Work out the finished part from the listing and answer in its coordinate system (mm). Face numbers are marked on the shaded views. A direction names the side the tool comes from. Round coordinates to 2 decimals unless told otherwise and drop trailing zeros. Order: outer loops, then holes, each group sorted by start corner. A loop starts at its lowest first (then second) coordinate and runs counter-clockwise, first axis right, second up. Notation, with made-up numbers: M 16,31 L 28,31 A16 ccw 28,57 Z; hole C 62,4 d1. An arc over 180 degrees is marked long. Return JSON: item names as keys, results as strings.
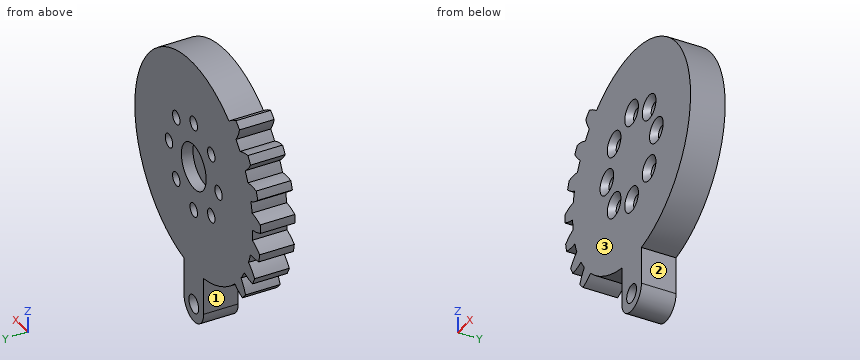
from build123d import *

# Parameters (mm, degrees)
SKETCH1_R                                       = 19.05
BOSS_EXTRUDE1_DEPTH                             = 6
SKETCH8_R                                       = 4
CUT_EXTRUDE4_DEPTH                              = 2
BOSS_EXTRUDE3_DEPTH                             = 6
CIRPATTERN2_DEPTH                               = 6
SKETCH4_R                                       = 1.5875
BOSS_EXTRUDE4_DEPTH                             = 6
CSK_FOR_M2_FLAT_HEAD_MACHINE_SCREW1_D           = 2.4
CSK_FOR_M2_FLAT_HEAD_MACHINE_SCREW1_CSINK_D     = 4.4
CSK_FOR_M2_FLAT_HEAD_MACHINE_SCREW1_CSINK_ANGLE = 90
CIRPATTERN3_COUNT                               = 8


# Read off the part's stored shape, not the designer's step: CirPattern2
with BuildPart() as part:
    # Sketch1 → Boss-Extrude1 (new body)
    with BuildSketch(Plane(origin=(0, 0, 0), x_dir=(1, 0, 0), z_dir=(0, 1, 0))):
        with Locations(Location((0, 0, 0), (0, 0, 270))):
            Circle(SKETCH1_R)
    extrude(amount=BOSS_EXTRUDE1_DEPTH)

    # Sketch8 → Cut-Extrude4 (cut)
    with BuildSketch(Plane.XZ.offset(-6)):
        with Locations(Location((0, 0, 0), (0, 0, 270))):
            Circle(SKETCH8_R)
    extrude(amount=CUT_EXTRUDE4_DEPTH, mode=Mode.SUBTRACT)

    # Sketch3 → Boss-Extrude3 (add)
    with BuildSketch(Plane(origin=(0, 0, 0), x_dir=(1, 0, 0), z_dir=(0, 1, 0))):
        with BuildLine():
            ThreePointArc((-18.32709122, 5.198098444), (-19.680979383, 5.197152008), (-21.013329851, 4.956618665))
            ThreePointArc((-21.013329851, 4.956618665), (-21.175154204, 4.212000052), (-21.310601203, 3.462134657))
            ThreePointArc((-21.310601203, 3.462134657), (-20.171718001, 2.730042376), (-18.921250622, 2.211057413))
            ThreePointArc((-18.921250622, 2.211057413), (-18.683959592, 3.716470634), (-18.32709122, 5.198098444))
        make_face()
    extrude(amount=BOSS_EXTRUDE3_DEPTH)

    # CirPattern2 outline → CirPattern2 (add)
    with BuildSketch(Plane(origin=(0, 0, 0), x_dir=(1, 0, 0), z_dir=(0, 1, 0))):
        with BuildLine():
            ThreePointArc((-17.704260875, 7.032897477), (-17.085425728, 8.425599549), (-16.357243856, 9.764377784))
            ThreePointArc((-16.357243856, 9.764377784), (-17.665244353, 10.113875638), (-19.014450689, 10.226375946))
            ThreePointArc((-19.014450689, 10.226375946), (-19.36348249, 9.549012822), (-19.688393689, 8.859754733))
            ThreePointArc((-19.688393689, 8.859754733), (-18.777796417, 7.857843228), (-17.704260875, 7.032897477))
        make_face()
        with BuildLine():
            ThreePointArc((-15.280755006, 11.375457202), (-14.322548335, 12.560537779), (-13.272677354, 13.665230916))
            ThreePointArc((-13.272677354, 13.665230916), (-14.445652113, 14.341355358), (-15.719768136, 14.799222606))
            ThreePointArc((-15.719768136, 14.799222606), (-16.232221443, 14.235276148), (-16.724454683, 13.653597166))
            ThreePointArc((-16.724454683, 13.653597166), (-16.104199039, 12.450145051), (-15.280755006, 11.375457202))
        make_face()
        with BuildLine():
            ThreePointArc((-11.375457197, -15.280755), (-12.560537774, -14.322548329), (-13.66523091, -13.272677349))
            ThreePointArc((-13.66523091, -13.272677349), (-14.341355358, -14.445652113), (-14.799222606, -15.719768136))
            ThreePointArc((-14.799222606, -15.719768136), (-14.235276148, -16.232221443), (-13.653597166, -16.724454683))
            ThreePointArc((-13.653597166, -16.724454683), (-12.450145051, -16.104199039), (-11.375457197, -15.280755))
        make_face()
        with BuildLine():
            ThreePointArc((-14.942798311, -11.81589093), (-15.839496111, -10.583612937), (-16.634821136, -9.28359982))
            ThreePointArc((-16.634821136, -9.28359982), (-17.59149541, -10.241612555), (-18.363526703, -11.353809363))
            ThreePointArc((-18.363526703, -11.353809363), (-17.95142893, -11.994761331), (-17.516969515, -12.620771728))
            ThreePointArc((-17.516969515, -12.620771728), (-16.193990063, -12.33312711), (-14.942798311, -11.81589093))
        make_face()
        with BuildLine():
            ThreePointArc((-17.491812414, -7.545793421), (-18.039018964, -6.123421813), (-18.470775793, -4.661860306))
            ThreePointArc((-18.470775793, -4.661860306), (-19.642804121, -5.339624026), (-20.676386801, -6.214107244))
            ThreePointArc((-20.676386801, -6.214107244), (-20.444221496, -6.939878056), (-20.18658934, -7.657004037))
            ThreePointArc((-20.18658934, -7.657004037), (-18.834241415, -7.72157295), (-17.491812414, -7.545793421))
        make_face()
        with BuildLine():
            ThreePointArc((-21.580185309, -0.650923987), (-21.543774153, -1.41205356), (-21.480526461, -2.171424174))
            ThreePointArc((-21.480526461, -2.171424174), (-20.190970338, -2.583806354), (-18.84878841, -2.761462559))
            ThreePointArc((-18.84878841, -2.761462559), (-19.009212486, -1.245929612), (-19.047977604, 0.277577285))
            ThreePointArc((-19.047977604, 0.277577285), (-20.355488193, -0.073748943), (-21.580185309, -0.650923987))
        make_face()
    extrude(amount=CIRPATTERN2_DEPTH)

    # Sketch4 → Boss-Extrude4 (add)
    with BuildSketch(Plane(origin=(0, 6, 0), x_dir=(1, 0, 0), z_dir=(0, 1, 0))):
        with BuildLine():
            Line((-3.175, 4.000000056), (3.175, 4.000000056))
            Line((3.175, 4.000000056), (3.175, 25.4))
            ThreePointArc((3.175, 25.4), (0, 28.575), (-3.175, 25.4))
            Line((-3.175, 25.4), (-3.175, 4.000000056))
        make_face()
        with Locations(Location((0, 25.4, 0), (0, 0, 270))):
            Circle(SKETCH4_R, mode=Mode.SUBTRACT)
    extrude(amount=-BOSS_EXTRUDE4_DEPTH)

    # CSK for M2 Flat Head Machine Screw1 (through all)
    with Locations(Plane.XZ):
        with Locations((0, -8)):
            csk_for_m2_flat_head_machine_screw1 = CounterSinkHole(CSK_FOR_M2_FLAT_HEAD_MACHINE_SCREW1_D / 2, CSK_FOR_M2_FLAT_HEAD_MACHINE_SCREW1_CSINK_D / 2, counter_sink_angle=CSK_FOR_M2_FLAT_HEAD_MACHINE_SCREW1_CSINK_ANGLE)

    # CirPattern3: CSK for M2 Flat Head Machine Screw1 ×8 about axis
    cirpattern3_axis = Axis((0, 0, 0), (0, 1, 0))
    for i in range(1, CIRPATTERN3_COUNT):
        add(csk_for_m2_flat_head_machine_screw1.rotate(cirpattern3_axis, i * 360 / CIRPATTERN3_COUNT), mode=Mode.SUBTRACT)


solid = part.part
Item 1: Find section A-A (x = 0). State how many separate pieces and enclosed holes the cut face has, plus the area to 3 significant figures.
Output:
{"separate pieces": "4", "enclosed holes": "0", "area": "220 mm^2"}
Item 2: Find section D-D (x = 13). Determine the outline of the cut face in (y, z).
Output:
{"outline": "M 0,-13.92 L 6,-13.92 L 6,13.92 L 0,13.92 Z"}
Item 3: Find section C-C (z = 14.5). Determine the outline of the cut face in (x, y).
Output:
{"outline": "M -14.37,0 L 12.36,0 L 12.36,6 L -14.37,6 Z"}
Item 4: Which of the six approach directions +Z, -Z, +X, -X, +Y, -Y give full straight-line access (tool end or side, diameter ignored) to the marked faces 1, 2 and 3?
Output:
{"face 1": "-Z, -X, +Y, -Y", "face 2": "-Z, +X, +Y, -Y", "face 3": "+Z, -Z, +X, -X, -Y"}
Item 5: Consider line 1 along X through (y, z) = (1.05, -25.5); line 2 along X through (y, z) = (4.6, -1); line 3 along X through (y, z) = (0.7, -6). Determine where each line is inside the solid, lowest interval first. Write a range as [from, to].
Output:
{"line 1": "x = [-3.17, -1.58], [1.58, 3.17]", "line 2": "x = [-19.02, -8.66], [-7.34, -3.87], [3.87, 7.34], [8.66, 19.02]", "line 3": "x = [-18.08, -7.12], [-4.2, 4.2], [7.12, 18.08]"}
Item 6: Each of these flat-tipped pins is pushed along its axis until it touches: pin 1 (1.8 mm diameter, centred on y = 3, z = -20.5, fed in from +X) (3 decimals); pin 2 (4 mm diameter, centred on x = 5.66, z = 5.66, fed in from -Y); pin 3 (3 mm diameter, centred on x = -8, z = 0, fed in from -Y); pin 4 (2 mm diameter, centred on x = -15.5, z = -1.5, fed in from -Y). Where does it stop, or does it pass through?
Output:
{"pin 1": "stops at x = 3.175", "pin 2": "stops at y = 0.2", "pin 3": "stops at y = 0.7", "pin 4": "stops at y = 0"}
